from build123d import *

# Parameters (mm, degrees)
BOSS_EXTRUDE1_DEPTH = 40
FILLET1_R           = 5
FILLET2_R           = 5
FILLET3_R           = 5


with BuildPart() as part:
    # Sketch1 → Boss-Extrude1 (new body)
    with BuildSketch(Plane(origin=(0, 0, 0), x_dir=(1, 0, 0), z_dir=(0, 1, 0))):
        Polygon((0, 0), (300, 0), (300, 40), (40, 40), (40, 300), (0, 300), (0, 40), align=None)
    extrude(amount=BOSS_EXTRUDE1_DEPTH)

    # Fillet1
    fillet1_edges = [part.edges().sort_by_distance(p)[0] for p in [
        (150, 40, 0),
    ]]
    fillet(fillet1_edges, radius=FILLET1_R)

    # Fillet2
    fillet2_edges = [part.edges().sort_by_distance(p)[0] for p in [
        (170, 40, -40),
        (40, 40, -170),
        (40, 0, -170),
        (150, 0, 0),
    ]]
    fillet(fillet2_edges, radius=FILLET2_R)

    # Fillet3
    fillet3_edges = [part.edges().sort_by_distance(p)[0] for p in [
        (0, 1.464466094, -1.464466094),
        (0, 20, 0),
        (0, 38.535533906, -1.464466094),
        (167.5, 0, -40),
        (0, 0, -152.5),
        (0, 40, -152.5),
    ]]
    fillet(fillet3_edges, radius=FILLET3_R)


solid = part.part
Verification items for the finished model (mm, model axes). A direction names the side the tool comes from. Give positions to 0.01 mm unless a question says otherwise; leave off trailing zeros. Write each loop counter-clockwise with the first axis right and the second up, starting at its lowest first coordinate (ties: lowest second). Pieces come first, ordered by that corner, then holes.
(1) Cross-section at C-C (y = 19). Enter the section's corners in (x, z).
(2) Access from +Z, -Z, +X, -X, +Y, -Y to the whole of each face (thin tool, end or side, straight path). Record for faces 4 (the face through (150, 20, 0)), 5 (the face through (172, 20, -40)).
(3) Gauge pin test, flat ends, axial feed: pin 1 (15 mm diameter, centred on x = 122.5, y = 20.5, fed in from -Z); pin 2 (9 mm diameter, centred on y = 23, z = -189, fed in from +X); pin 3 (10 mm diameter, centred on y = 35.5, z = -156.5, fed in from -X). Record the tip position at first contact, or that the pin passes through.
(4) Mould release check, pull along X, two halves, no side actions. Record for faces 1 (the face through (0, 20, -155)), 2 (the face through (300, 20, -20)), 3 (the face through (86, 0, -33)): +X half, -X half, draft (parallel to the pull), parting line (faces both ways), or undercut.
(5) Cross-section at A-A (x = 226.5). Enter the section's corners in (y, z).
(6) Material ranges on line 1 (Z direction, x = 261.5, y = 35); line 2 (X direction, y = 7, z = -98.5); line 3 (Z direction, x = 222, y = 3), recorded low to high.
(7) Cross-section at B-B (z = -280). Enter the section's corners in (x, y), plus the area to 3 significant figures.
Worked out:
1. outline: (0, -300) - (40, -300) - (40, -40) - (300, -40) - (300, 0) - (5, 0) arc R5 ccw to (0, -5) - close
2. face 4: +Z, +X, -X, +Y, -Y
2. face 5: -Z, +X, +Y, -Y
3. pin 1: stops at z = -40
3. pin 2: stops at x = 40
3. pin 3: stops at x = 0
4. face 1: -X half
4. face 2: +X half
4. face 3: draft
5. outline: (0, -35) arc R5 ccw to (5, -40) - (35, -40) arc R5 ccw to (40, -35) - (40, -5) arc R5 ccw to (35, 0) - (5, 0) arc R5 ccw to (0, -5) - close
6. line 1: z = -40 to 0
6. line 2: x = 0 to 40
6. line 3: z = -39.58 to -0.42
7. outline: (0, 5) arc R5 ccw to (5, 0) - (35, 0) arc R5 ccw to (40, 5) - (40, 35) arc R5 ccw to (35, 40) - (5, 40) arc R5 ccw to (0, 35) - close
7. area: 1,580 mm2
